The drawing under review shows one solid part. Ordinate dimensions are in mm from its lowest x, y, z. A direction names the side the tool comes from. Coordinates: 2 decimals unless noted, no trailing zeros. Write each loop counter-clockwise with the first axis right and the second up, starting at its lowest first coordinate (ties: lowest second). Pieces come first, ordered by that corner, then holes.
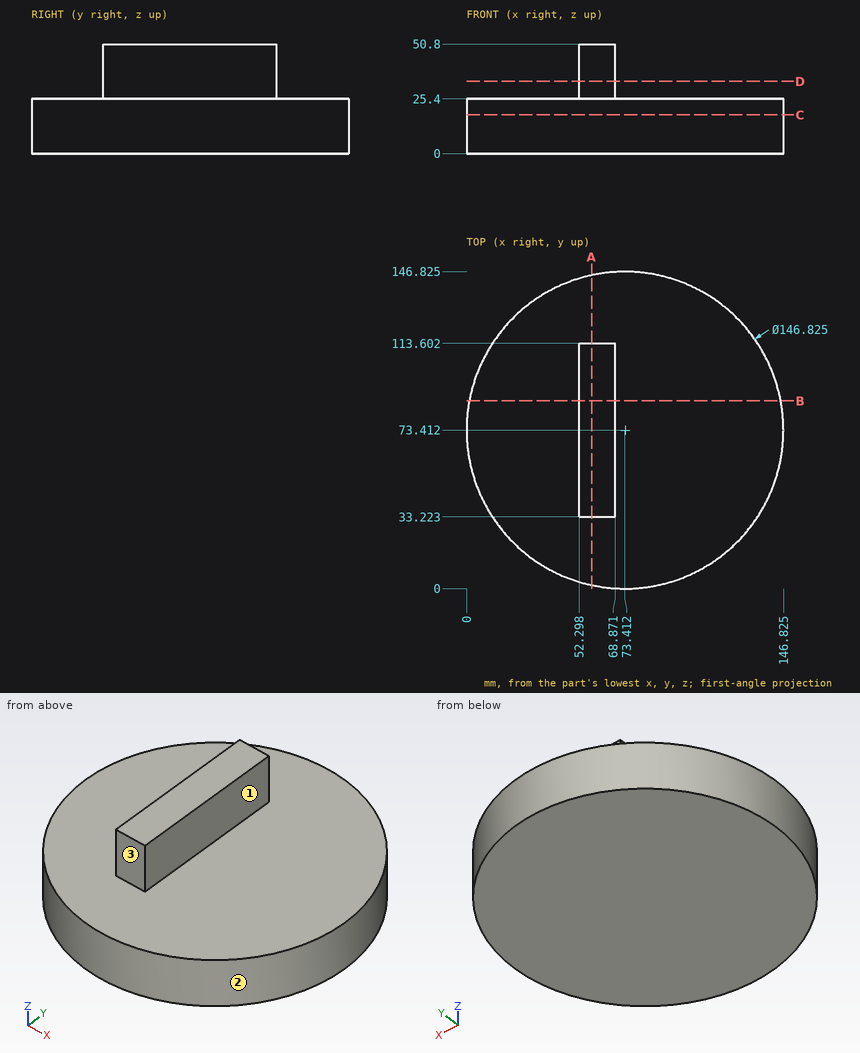
1) Tool access review of the marked faces 1, 2 and 3: name each direction out of +Z, -Z, +X, -X, +Y, -Y from which nothing blocks a thin tool from reaching the whole face with its end or side.
2) Clearance check with flat-ended pins moving along their axes: P1, Ø2, axis at y = 102, z = 42, coming from the -X side; P2, Ø18, axis at x = 59.5, z = 36, coming from the -Y side; P3, Ø12, axis at x = 102, z = 18, coming from the +Y side; P4, Ø6, axis at x = 94.5, z = 28.5, coming from the -Y side. State where each tip first meets the part, or that it passes through.
3) Consider section B-B (y = 87). Give the boundary of the cut face in (x, z).
4) Consider section C-C (z = 18). Give the boundary of the cut face in (x, y) (1 decimal).
5) Consider section A-A (x = 58). Give the boundary of the cut face in (y, z).
6) Consider section D-D (z = 33.5). Give the boundary of the cut face in (x, y).
7) For L1, parallel to Z at x = 23.5, y = 127; L2, parallel to X at y = 54, z = 32; L3, parallel to X at y = 137.5, z = 17.5 (1 decimal), list the stretches that pass through material, from the lowest coordinate up.
Results:
1. face 1: +Z, +X, +Y, -Y
1. face 2: +Z, -Z
1. face 3: +Z, +X, -X, -Y
2. P1: stops at x = 52.3
2. P2: stops at y = 33.22
2. P3: stops at y = 143.26
2. P4: passes through
3. outline: (1.27, 0) - (145.56, 0) - (145.56, 25.4) - (68.87, 25.4) - (68.87, 50.8) - (52.3, 50.8) - (52.3, 25.4) - (1.27, 25.4) - close
4. outline: circle Ø146.8 at (73.4, 73.4)
5. outline: (1.64, 0) - (145.19, 0) - (145.19, 25.4) - (113.6, 25.4) - (113.6, 50.8) - (33.22, 50.8) - (33.22, 25.4) - (1.64, 25.4) - close
6. outline: (52.3, 33.22) - (68.87, 33.22) - (68.87, 113.6) - (52.3, 113.6) - close
7. L1: z = 0 to 25.4
7. L2: x = 52.3 to 68.87
7. L3: x = 37.6 to 109.2
